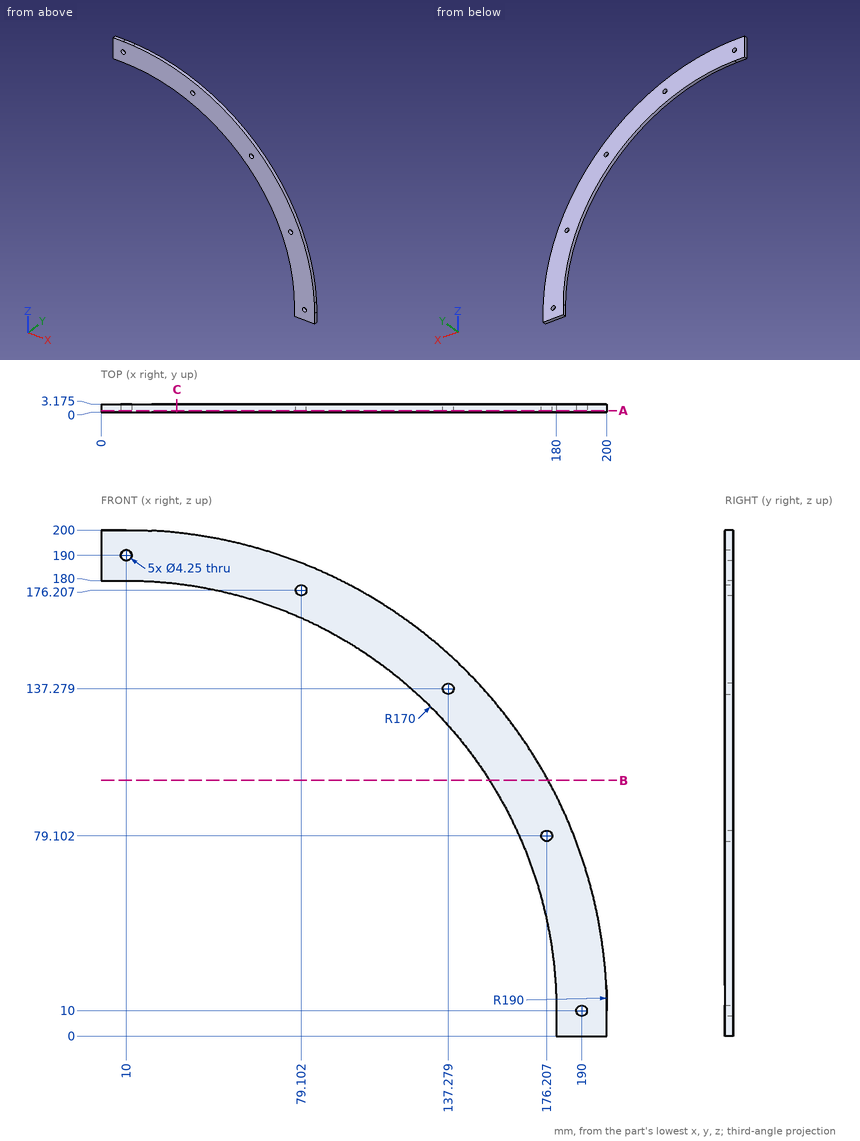
The drawing under review shows one solid part. Ordinate dimensions are in mm from its lowest x, y, z. Coordinates: 2 decimals unless noted, no trailing zeros. Write each loop counter-clockwise with the first axis right and the second up, starting at its lowest first coordinate (ties: lowest second). Pieces come first, ordered by that corner, then holes. Notation, with made-up numbers: (20.5, -18.5) - (79.5, -18.5) arc R15 cw to (79.5, -10.5) - close; hole circle Ø6 at (15.5, 16). An arc over 180 degrees is marked (long way). Answer in a Markdown table with one row per item. Add a question column.
Q1. For P1, Ø7, axis at x = 176.21, z = 79.1, coming from the +Y side (3 decimals); P2, Ø4, axis at x = 10, z = 190, coming from the -Y side; P3, Ø1.5, axis at x = 117, y = 1, coming from the -Z side; P4, Ø1, axis at x = 158.5, y = 0.5, coming from the +Z side (1 decimal), all flat-tipped, find the tip position at first contact; note any pin that passes through.
Q2. We need section C-C, the plane x = 30. State the section outline as (y, z) points (1 decimal), and give its area (3 significant figures).
Q3. For probe 1 along X at (y, z) = (1.05, 10) (1 decimal); probe 2 along X at (y, z) = (2.7, 165) (1 decimal), list the stretches that pass through material, from the lowest coordinate up.
Q4. We need section B-B, the plane z = 101. State the section outline as (x, y) points (1 decimal).
Q5. We need section A-A, the plane y = 0.55. Count the separate pieces of the cut face and the enclosed holes in it, and give its area (3 significant figures).
Answer list:
| question | item | result |
|---|---|---|
| 1 | P1 | stops at y = 3.175 |
| 1 | P2 | passes through |
| 1 | P3 | stops at z = 141.49 |
| 1 | P4 | stops at z = 129.1 |
| 2 | outline | (0, 178.8) - (3.2, 178.8) - (3.2, 198.9) - (0, 198.9) - close |
| 2 | area | 63.9 mm2 |
| 3 | probe 1 | x = 180 to 187.9, 192.1 to 200 |
| 3 | probe 2 | x = 79.8 to 119.9 |
| 4 | outline | (153.6, 0) - (176.8, 0) - (176.8, 3.2) - (153.6, 3.2) - close |
| 5 | separate pieces | 1 |
| 5 | enclosed holes | 5 |
| 5 | area | 5,980 mm2 |
